Input: part model. Units: mm. Frame: model coordinates. A direction names the side the tool comes from. Coordinates: 2 decimals unless noted, no trailing zeros. Order: outer loops, then holes, each group sorted by start corner. A loop starts at its lowest first (then second) coordinate and runs counter-clockwise, first axis right, second up. Notation, with made-up numbers: (14.5, 39.5) -> (50.5, 39.5) arc R9 cw to (50.5, 50.5) -> close; hole circle Ø11 at (78.25, 36). An arc over 180 degrees is marked (long way). One line per question, with ' | ' between items.
```python
from build123d import *

# Parameters (mm, degrees)
SKETCH1_R           = 5
BOSS_EXTRUDE1_DEPTH = 560
SKETCH2_R           = 10
BOSS_EXTRUDE2_DEPTH = 10
SKETCH3_R           = 10
BOSS_EXTRUDE3_DEPTH = 10


with BuildPart() as part:
    # Sketch1 → Boss-Extrude1 (new body)
    with BuildSketch(Plane(origin=(0, 0, 0), x_dir=(0, 0, -1), z_dir=(1, 0, 0))):
        Circle(SKETCH1_R)
    extrude(amount=BOSS_EXTRUDE1_DEPTH)

    # Sketch2 → Boss-Extrude2 (add)
    with BuildSketch(Plane(origin=(560, 0, 0), x_dir=(0, 0, -1), z_dir=(1, 0, 0))):
        Circle(SKETCH2_R)
    extrude(amount=BOSS_EXTRUDE2_DEPTH)

    # Sketch3 → Boss-Extrude3 (add)
    with BuildSketch(Plane.ZY):
        Circle(SKETCH3_R)
    extrude(amount=BOSS_EXTRUDE3_DEPTH)


solid = part.part
```
1. Cut plane C-C, the plane x = 62. Return loops of the section in (y, z), and give its area (3 significant figures).
Recorded:
outline: circle Ø10 at (0, 0) | area: 78.5 mm^2
2. Mould query, pull axis X, two halves, no side actions, for faces 1 (the face through (-10, 0, 0)), 2 (the face through (0, -2, -5)), 3 (the face through (-4.93, -9.76, -2.17)). Classes: released by +X, released by -X, zero draft, split by the parting line, or undercut.
Recorded:
face 1: released by -X | face 2: undercut | face 3: zero draft
3. Cut plane A-A, the plane z = 0. Return loops of the section in (x, y).
Recorded:
outline: (-10, -10) -> (0, -10) -> (0, -5) -> (560, -5) -> (560, -10) -> (570, -10) -> (570, 10) -> (560, 10) -> (560, 5) -> (0, 5) -> (0, 10) -> (-10, 10) -> close
4. Ray query, line 1 (X direction, y = -7, z = -2.75); line 2 (Y direction, x = 482.5, z = 1); line 3 (Y direction, x = 336.5, z = -0.25). Return the intervals inside material, ascending. Write a range as [from, to].
Recorded:
line 1: x = [-10, 0], [560, 570] | line 2: y = [-4.9, 4.9] | line 3: y = [-4.99, 4.99]
5. Pin query (flat end, axial travel): pin 1 Ø4 at (x, z) = (369.5, -8) entering from +Y; pin 2 Ø2 at (x, y) = (505.5, 1.5) entering from -Z; pin 3 Ø5 at (x, y) = (199, -1.5) entering from +Z; pin 4 Ø10 at (x, z) = (63.5, 2.5) entering from +Y. Return the tip coordinate at first contact, or that it passes through.
Recorded:
pin 1: passes through | pin 2: stops at z = -4.97 | pin 3: stops at z = 5 | pin 4: stops at y = 5
6. Access query for faces 4 (the face through (560, -2, 5)), 5 (the face through (564.93, -9.76, 2.17)). Directions: +Z, -Z, +X, -X, +Y, -Y. A direction counts if a zero-diameter tool reaches every point of the face in a straight line with its end or side. Return the directions, or none.
Recorded:
face 4: none | face 5: +X, -X
